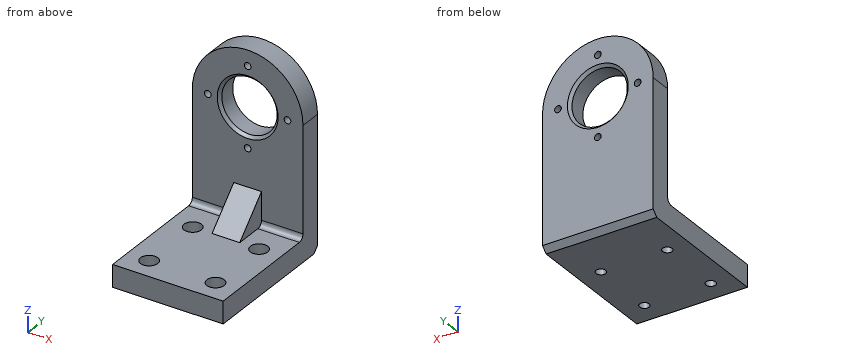
```python
from build123d import *

# Parameters (mm, degrees)
F0_R            = 50
F1_DEPTH        = 40
F2_SIZE         = 5
F3_D            = 12.1
F4_DEPTH        = 260
F5_R            = 10
F6_SIZE         = 10
F8_DEPTH        = 25
F10_D           = 17.5
F10_CBORE_D     = 31.5
F10_CBORE_DEPTH = 20


with BuildPart() as f1:
    # F0 (on Front) → F1 (new body)
    with BuildSketch(Plane.XZ):
        with BuildLine():
            Line((-100, 0), (0, 0))
            Line((0, 0), (100, 0))
            Line((100, 0), (100, 200))
            ThreePointArc((100, 200), (0, 300), (-100, 200))
            Line((-100, 200), (-100, 0))
        make_face()
        with Locations((0, 200)):
            Circle(F0_R, mode=Mode.SUBTRACT)
        Polygon((100, 0), (0, 0), (-100, 0), (-100, -40), (100, -40), align=None)
    extrude(amount=F1_DEPTH)

    # F2
    f2_edges = [f1.edges().sort_by_distance(p)[0] for p in [
        (50, -20, 200),
        (-50, 0, 200),
        (-50, -40, 200),
    ]]
    chamfer(f2_edges, length=F2_SIZE)

    # F3 (through all)
    with Locations(Plane(origin=(0, 0, 0), x_dir=(1, 0, 0), z_dir=(0, 1, 0))):
        with Locations((0, -272), (72, -200), (0, -128), (-72, -200)):
            Hole(F3_D / 2)

    # F0 (on Front) → F4 (join)
    with BuildSketch(Plane.XZ):
        Polygon((100, 0), (0, 0), (-100, 0), (-100, -40), (100, -40), align=None)
    extrude(amount=F4_DEPTH)

    # F5
    f5_edges = [f1.edges().sort_by_distance(p)[0] for p in [
        (0, -40, 0),
    ]]
    fillet(f5_edges, radius=F5_R)

    # F6
    f6_edges = [f1.edges().sort_by_distance(p)[0] for p in [
        (0, 0, -40),
    ]]
    chamfer(f6_edges, length=F6_SIZE)

    # F7 (on Right) → F8 (join, symmetric)
    with BuildSketch(Plane.YZ):
        with BuildLine():
            ThreePointArc((-50, 0), (-42.9289321881, 2.9289321881), (-40, 10))
            Line((-40, 10), (-40, 60))
            Line((-40, 60), (-100, 0))
            Line((-100, 0), (-50, 0))
        make_face()
    extrude(amount=F8_DEPTH, both=True)

    # F10 (through all)
    with Locations(Plane.XY):
        with Locations((-60, -100), (60, -100), (60, -220), (-60, -220)):
            CounterBoreHole(F10_D / 2, F10_CBORE_D / 2, F10_CBORE_DEPTH)


solid = f1.part
```
Source: CAD feature listing. Evaluate the final solid. Frame: model axes, mm. Coordinates: 2 decimals unless noted, no trailing zeros. Write each loop counter-clockwise with the first axis right and the second up, starting at its lowest first coordinate (ties: lowest second). Pieces come first, ordered by that corner, then holes. Notation, with made-up numbers: (39, 26) - (76, 26) arc R13 ccw to (76, 31) - close; hole circle Ø1 at (1.25, -31.75). An arc over 180 degrees is marked (long way). Answer as a JSON object with one key per item and string values.
Q1. Section query C-C, the plane y = -72. Output: boundary loops of the cut face in (x, z).
Ans:
{"outline": "(-100, -40) - (100, -40) - (100, 0) - (25, 0) - (25, 28) - (-25, 28) - (-25, 0) - (-100, 0) - close"}
Q2. Section query B-B, the plane x = 60. Output: boundary loops of the cut face in (y, z).
Ans:
{"outline": "(-260, -40) - (-228.75, -40) - (-228.75, -20) - (-235.75, -20) - (-235.75, 0) - (-260, 0) - close; (-211.25, -40) - (-108.75, -40) - (-108.75, -20) - (-115.75, -20) - (-115.75, 0) - (-204.25, 0) - (-204.25, -20) - (-211.25, -20) - close; (-91.25, -40) - (-10, -40) - (0, -30) - (0, 280) - (-40, 280) - (-40, 10) arc R10 cw to (-50, 0) - (-84.25, 0) - (-84.25, -20) - (-91.25, -20) - close"}
Q3. Section query A-A, the plane z = 128. Output: boundary loops of the cut face in (x, y).
Ans:
{"outline": "(-100, -40) - (-6.05, -40) - (-6.05, 0) - (-100, 0) - close; (6.05, -40) - (100, -40) - (100, 0) - (6.05, 0) - close"}
Q4. Section query D-D, the plane z = 28.5. Output: boundary loops of the cut face in (x, y), plus the area to 4 significant figures.
Ans:
{"outline": "(-100, -40) - (-25, -40) - (-25, -71.5) - (25, -71.5) - (25, -40) - (100, -40) - (100, 0) - (-100, 0) - close", "area": "9,575 mm2"}
Q5. Material intervals for line 1 (Z direction, x = 0, y = -12); line 2 (Y direction, x = -60, z = -13); line 3 (Y direction, x = 60, z = -28), sorted ascending. Write a range as [from, to].
Ans:
{"line 1": "z = [-40, 121.95], [134.05, 150], [250, 265.95], [278.05, 300]", "line 2": "y = [-260, -235.75], [-204.25, -115.75], [-84.25, 0]", "line 3": "y = [-260, -228.75], [-211.25, -108.75], [-91.25, 0]"}
Q6. First-contact query: pin 1 Ø14 at (x, z) = (-72, 200) entering from -Y; pin 2 Ø2 at (x, y) = (-18.5, -107) entering from +Z; pin 3 Ø23 at (x, y) = (-60, -220) entering from +Z. Flat tips, straight axial feed; report the tip coordinate or a pass-through.
Ans:
{"pin 1": "stops at y = -40", "pin 2": "stops at z = 0", "pin 3": "stops at z = -20"}
